from build123d import *

# Parameters (mm, degrees)
BOSS_EXTRUDE1_DEPTH = 50
SKETCH2_R           = 30
BOSS_EXTRUDE2_DEPTH = 75
SKETCH3_R           = 18.435978865
BOSS_EXTRUDE3_DEPTH = 30
SKETCH4_R           = 10
CUT_EXTRUDE1_DEPTH  = 220
FILLET1_R           = 1
SKETCH6_R           = 10
CUT_EXTRUDE3_DEPTH  = 110


with BuildPart() as part:
    # Sketch1 → Boss-Extrude1 (new body)
    with BuildSketch(Plane(origin=(0, 0, 0), x_dir=(1, 0, 0), z_dir=(0, 1, 0))):
        Polygon((-42.485875706, 40.677966102), (-42.485875706, -8.276836158), (-62.824858757, -8.276836158), (-62.824858757, -39.011299435), (-62.824858757, -70.484281789), (-47.824858757, -70.484281789), (-47.824858757, -19.011299435), (-32.824858757, -19.011299435), (-32.824858757, 15.988700565), (7.514124294, 15.988700565), (7.514124294, -19.011299435), (22.514124294, -19.011299435), (22.514124294, -70.484281789), (37.514124294, -70.484281789), (37.514124294, -39.011299435), (37.514124294, -1.511299435), (22.514124294, -1.511299435), (22.514124294, 46.553672316), (-42.485875706, 46.553672316), align=None)
    extrude(amount=BOSS_EXTRUDE1_DEPTH)

    # Sketch2 → Boss-Extrude2 (add, symmetric)
    with BuildSketch(Plane(origin=(0, 50, 0), x_dir=(1, 0, 0), z_dir=(0, 1, 0))):
        with Locations((-9.985875706, 61.810417825)):
            Circle(SKETCH2_R)
    extrude(amount=BOSS_EXTRUDE2_DEPTH, both=True)

    # Sketch3 → Boss-Extrude3 (add)
    with BuildSketch(Plane(origin=(0, 125, 0), x_dir=(1, 0, 0), z_dir=(0, 1, 0))):
        with Locations((-9.985875706, 61.810417825)):
            Circle(SKETCH3_R)
    extrude(amount=BOSS_EXTRUDE3_DEPTH)

    # Sketch4 → Cut-Extrude1 (cut)
    with BuildSketch(Plane(origin=(0, 155, 0), x_dir=(1, 0, 0), z_dir=(0, 1, 0))):
        with Locations((-9.985875706, 61.810417825)):
            Circle(SKETCH4_R)
    extrude(amount=-CUT_EXTRUDE1_DEPTH, mode=Mode.SUBTRACT)

    # Fillet1
    fillet1_edges = [part.edges().sort_by_distance(p)[0] for p in [
        (30.014124294, 0, 70.484281789),
        (-55.324858757, 0, 70.484281789),
        (-55.324858757, 50, 70.484281789),
        (30.014124294, 50, 70.484281789),
    ]]
    fillet(fillet1_edges, radius=FILLET1_R)

    # Sketch6 → Cut-Extrude3 (cut, symmetric)
    with BuildSketch(Plane(origin=(-47.824858757, 0, 0), x_dir=(0, 0, -1), z_dir=(1, 0, 0))):
        with Locations((-44.247790612, 25)):
            Circle(SKETCH6_R)
    extrude(amount=CUT_EXTRUDE3_DEPTH, both=True, mode=Mode.SUBTRACT)


solid = part.part
Check sheet for the modelled part. Datum: model origin and axes. Units: mm. A direction names the side the tool comes from. Give positions to 0.01 mm unless a question says otherwise; leave off trailing zeros. Write each loop counter-clockwise with the first axis right and the second up, starting at its lowest first coordinate (ties: lowest second). Pieces come first, ordered by that corner, then holes. Notation, with made-up numbers: (60, 5) -> (77, 5) arc R30 ccw to (77, 32) -> close; hole circle Ø8 at (16.5, 2.25). An arc over 180 degrees is marked (long way). Write item = value, one per line.
Item 1: Tool access check on faces 4 (the flat face through (-24, 125, -49)), 5 (the flat face through (7.514, 25, 1)), 6 (the flat face through (30, 25, 1.511)), 7 (the flat face through (-55, 25, 70.484)). Record the directions out of +Z, -Z, +X, -X, +Y, -Y that give a thin tool (end or side, any length) a straight path to the whole face; none if there is none.
Output:
face_4 = +Y
face_5 = +Z, +Y, -Y
face_6 = -Z, +X, +Y, -Y
face_7 = +Z, +X, -X, +Y, -Y
Item 2: Gauge pin test, flat ends, axial feed: pin 1 (6 mm diameter, centred on y = 131, z = -42.5, fed in from -X); pin 2 (22.5 mm diameter, centred on x = -54, y = 17, fed in from -Z); pin 3 (15 mm diameter, centred on y = 21, z = 41, fed in from -X); pin 4 (3 mm diameter, centred on x = -17, y = 50, fed in from +Z). Record the tip position at first contact, or that the pin passes through.
Output:
pin_1 = -18.58
pin_2 = 8.28
pin_3 = -62.82
pin_4 = -15.99
Item 3: Scan lines: probe 1 along Z at (x, y) = (-9.5, 2); probe 2 along X at (y, z) = (135.5, -61.5); probe 3 along Z at (x, y) = (-51, 43). Record each from-to range of solid material in increasing order. Write a range as from..to.
Output:
probe_1 = -91.81..-71.8, -51.82..-15.99
probe_2 = -28.42..-19.98, 0.01..8.45
probe_3 = 8.28..70.48
Item 4: Sectioned sample at B-B on y = 25. Record the boundary of the cut face in (x, z), and give its area (3 significant figures).
Output:
outline = (-62.82, 8.28) -> (-42.49, 8.28) -> (-42.49, -46.55) -> (-35.82, -46.55) arc R30 ccw (long way) to (15.84, -46.55) -> (22.51, -46.55) -> (22.51, 1.51) -> (37.51, 1.51) -> (37.51, 34.25) -> (22.51, 34.25) -> (22.51, 19.01) -> (7.51, 19.01) -> (7.51, -15.99) -> (-32.82, -15.99) -> (-32.82, 19.01) -> (-47.82, 19.01) -> (-47.82, 34.25) -> (-62.82, 34.25) -> close; (-62.82, 54.25) -> (-47.82, 54.25) -> (-47.82, 70.48) -> (-62.82, 70.48) -> close; (22.51, 54.25) -> (37.51, 54.25) -> (37.51, 70.48) -> (22.51, 70.48) -> close; hole circle Ø20 at (-9.99, -61.81)
area = 6,250 mm^2
Item 5: Sectioned sample at A-A on z = 28.5. Record the boundary of the cut face in (x, y), and give its area (3 significant figures).
Output:
outline = (-62.82, 0) -> (-47.82, 0) -> (-47.82, 50) -> (-62.82, 50) -> close; (22.51, 0) -> (37.51, 0) -> (37.51, 50) -> (22.51, 50) -> close
area = 1,500 mm^2
Item 6: Sectioned sample at D-D on y = 143. Record the boundary of the cut face in (x, z), and give its area (3 significant figures).
Output:
outline = circle Ø36.87 at (-9.99, -61.81); hole circle Ø20 at (-9.99, -61.81)
area = 754 mm^2
Item 7: Sectioned sample at C-C on y = 81. Record the boundary of the cut face in (x, z).
Output:
outline = circle Ø60 at (-9.99, -61.81); hole circle Ø20 at (-9.99, -61.81)
Item 8: Release check for a two-part mould opening along Y. For faces 1 (the flat face through (9, 50, 11)), 2 (the flat face through (-42.486, 25, -20)), 3 (the cylindrical face through (30.12, 28, 34.71)) record: +Y half, -Y half, draft (parallel to the pull), parting line (faces both ways), or undercut.
Output:
face_1 = +Y half
face_2 = draft
face_3 = undercut
